Part model, mm, in its own coordinate system. A direction names the side the tool comes from. Round coordinates to 2 decimals unless told otherwise and drop trailing zeros. Order: outer loops, then holes, each group sorted by start corner. A loop starts at its lowest first (then second) coordinate and runs counter-clockwise, first axis right, second up. Notation, with made-up numbers: (-9, 50.5) -> (-3, 50.5) arc R19 ccw to (-3, 62.5) -> close; hole circle Ø9 at (-28, -12.75). An arc over 180 degrees is marked (long way). Answer as a JSON object with one key per item and string values. Group by question number.
```python
from build123d import *

# Parameters (mm, degrees)
SKETCH_1_W          = 2
SKETCH_1_H          = 8
EXTRUDE_2_DEPTH     = 8
EXTRUDE_2_2_DEPTH   = 8
SKETCH_1_3_R        = 7.129483457
EXTRUDE_3_DEPTH     = 150
SKETCH_2_W          = 2
SKETCH_2_H          = 8
EXTRUDE_4_DEPTH     = 10
FILLET_2_R          = 2
FILLET_3_R          = 2
FILLET_4_R          = 2
FILLET_5_R          = 2
SKETCH_3_R          = 3
CUT_EXTRUDE_1_DEPTH = 10
EXTRUDE_START       = 20
EXTRUDE_5_DEPTH     = 20
SKETCH_5_W          = 8
SKETCH_5_H          = 11.5
EXTRUDE_6_DEPTH     = 20
FILLET_6_R          = 3
FILLET_7_R          = 3
SKETCH_6_R          = 3
CUT_EXTRUDE_2_DEPTH = 20


with BuildPart() as part:
    # Sketch 1 → Extrude 2 (new body)
    with BuildSketch(Plane.XY):
        with Locations((-3, 0)):
            Rectangle(SKETCH_1_W, SKETCH_1_H)
    extrude(amount=EXTRUDE_2_DEPTH)



with BuildPart() as body_2:
    # Sketch 1 → Extrude 2 2 (new body)
    with BuildSketch(Plane.XY):
        with Locations((3, 0)):
            Rectangle(SKETCH_1_W, SKETCH_1_H)
    extrude(amount=EXTRUDE_2_2_DEPTH)


with BuildPart() as part_1:
    add(part.part)

    add(body_2.part)  # Extrude 3 merges body 2
    # Sketch 1_3 → Extrude 3 (add)
    with BuildSketch(Plane.XY):
        Circle(SKETCH_1_3_R)
    extrude(amount=-EXTRUDE_3_DEPTH)

    # Sketch 2 → Extrude 4 (add)
    with BuildSketch(Plane.XY.offset(8)):
        with Locations((3, 0)):
            Rectangle(SKETCH_2_W, SKETCH_2_H)
        with Locations((-3, 0)):
            Rectangle(SKETCH_2_W, SKETCH_2_H)
    extrude(amount=EXTRUDE_4_DEPTH)

    # Fillet 2
    fillet_2_edges = [part_1.edges().sort_by_distance(p)[0] for p in [
        (-3, -4, 18),
    ]]
    fillet(fillet_2_edges, radius=FILLET_2_R)

    # Fillet 3
    fillet_3_edges = [part_1.edges().sort_by_distance(p)[0] for p in [
        (3, -4, 18),
    ]]
    fillet(fillet_3_edges, radius=FILLET_3_R)

    # Fillet 4
    fillet_4_edges = [part_1.edges().sort_by_distance(p)[0] for p in [
        (-3, 4, 18),
    ]]
    fillet(fillet_4_edges, radius=FILLET_4_R)

    # Fillet 5
    fillet_5_edges = [part_1.edges().sort_by_distance(p)[0] for p in [
        (3, 4, 18),
    ]]
    fillet(fillet_5_edges, radius=FILLET_5_R)

    # Sketch 3 → Cut-Extrude 1 (cut)
    with BuildSketch(Plane.ZY.offset(4)):
        with Locations((13.5, 0.200340445)):
            Circle(SKETCH_3_R)
    extrude(amount=-CUT_EXTRUDE_1_DEPTH, mode=Mode.SUBTRACT)

    # Sketch 4 → Extrude 5 (add)
    with BuildSketch(Plane.XY.offset(EXTRUDE_START)):
        with BuildLine():
            Line((-4, -4), (-4, 0))
            Line((-4, 0), (-4, 4))
            Line((-4, 4), (-4, 5.901655223))
            ThreePointArc((-4, 5.901655223), (-7.129483457, 0), (-4, -5.901655223))
            Line((-4, -5.901655223), (-4, -4))
        make_face()
        with BuildLine():
            ThreePointArc((7.129483457, 0), (6.298708923, 3.34002998), (4, 5.901655223))
            Line((4, 5.901655223), (4, 4))
            Line((4, 4), (4, 0))
            Line((4, 0), (4, -4))
            Line((4, -4), (4, -5.901655223))
            ThreePointArc((4, -5.901655223), (6.298708923, -3.34002998), (7.129483457, 0))
        make_face()
    extrude(amount=-EXTRUDE_5_DEPTH)

    # Sketch 5 → Extrude 6 (add)
    with BuildSketch(Plane(origin=(0, 0, -150), x_dir=(-1, 0, 0), z_dir=(0, 0, -1))):
        Rectangle(SKETCH_5_W, SKETCH_5_H)
    extrude(amount=EXTRUDE_6_DEPTH)

    # Fillet 6
    fillet_6_edges = [part_1.edges().sort_by_distance(p)[0] for p in [
        (0, -5.75, -170),
    ]]
    fillet(fillet_6_edges, radius=FILLET_6_R)

    # Fillet 7
    fillet_7_edges = [part_1.edges().sort_by_distance(p)[0] for p in [
        (0, 5.75, -170),
    ]]
    fillet(fillet_7_edges, radius=FILLET_7_R)

    # Sketch 6 → Cut-Extrude 2 (cut)
    with BuildSketch(Plane(origin=(4, 0, 0), x_dir=(0, 0, -1), z_dir=(1, 0, 0))):
        with Locations((165, 0)):
            Circle(SKETCH_6_R)
    extrude(amount=-CUT_EXTRUDE_2_DEPTH, mode=Mode.SUBTRACT)


solid = part_1.part
```
Q1. Drop flat-ended pins along their axis: pin 1 Ø5 at (x, z) = (-4.5, -134) entering from +Y; pin 2 Ø0.6 at (x, z) = (3, 7.5) entering from -Y; pin 3 Ø6 at (x, z) = (-4.5, -44) entering from +Y. Give the stop position or say it passes through.
Q2. Band-saw the part on B-B (x = 0). List the corners of the cut face in (y, z).
Q3. Band-saw the part on C-C (z = -165). List the corners of the cut face in (x, y), plus the area to 3 significant figures.
Q4. Wall check: line 1 (Y direction, x = -1.5, z = -165); line 2 (Y direction, x = -2.6, z = 13.5); line 3 (X direction, y = -0.25, z = -152). Give the ranges that are in metal, low to high. Write a range as [from, to].
Q5. Band-saw the part on A-A (z = 13.5). List the corners of the cut face in (x, y), plus the area to 3 significant figures.
Q6. Band-saw the part on D-D (z = -34). List the corners of the cut face in (x, y).
Q7. Two-plate mould, pull along X, no slides. Class faces 4 (the flat face through (-4, 0, -160)), 5 (the flat face through (4, 0, 14)), 6 (the flat face through (0, 5.75, -158)): +X half, -X half, draft (parallel to the pull), parting line (faces both ways), or undercut.
Q8. Which spindle directions (+Z, -Z, +X, -X, +Y, -Y) get a long thin tool onto all of the face, cutting with end or side? Do faces 1 (the flat face through (2, 0, 7)), 2 (the flat face through (4, 5, 12)), 3 (the cylindrical face through (-3, 0.3, 10.5)). Say none if no direction does.
Completed:
{
 "1": {"pin 1": "y = 6.84", "pin 2": "y = -4", "pin 3": "y = 6.97"},
 "2": {"outline": "(-7.13, -150) -> (-5.75, -150) -> (-5.75, -167) arc R3 ccw to (-2.75, -170) -> (2.75, -170) arc R3 ccw to (5.75, -167) -> (5.75, -150) -> (7.13, -150) -> (7.13, 0) -> (-7.13, 0) -> close; hole circle Ø6 at (0, -165)"},
 "3": {"outline": "(-4, -5.75) -> (4, -5.75) -> (4, -3) -> (-4, -3) -> close; (-4, 3) -> (4, 3) -> (4, 5.75) -> (-4, 5.75) -> close", "area": "44.0 mm2"},
 "4": {"line 1": "[-5.75, -3], [3, 5.75]", "line 2": "[-4, -2.8], [3.2, 4]", "line 3": "[-4, 4]"},
 "5": {"outline": "(-4, -5.9) -> (-4, -4) -> (-2, -4) -> (-2, -2.8) -> (-4, -2.8) -> (-4, 3.2) -> (-2, 3.2) -> (-2, 4) -> (-4, 4) -> (-4, 5.9) arc R7.13 ccw to start; (2, -4) -> (4, -4) -> (4, -5.9) arc R7.13 ccw to (4, 5.9) -> (4, 4) -> (2, 4) -> (2, 3.2) -> (4, 3.2) -> (4, -2.8) -> (2, -2.8) -> close", "area": "59.9 mm2"},
 "6": {"outline": "circle Ø14.26 at (0, 0)"},
 "7": {"face 4": "-X half", "face 5": "undercut", "face 6": "draft"},
 "8": {"face 1": "+Z, +Y, -Y", "face 2": "+Z", "face 3": "none"}
}
